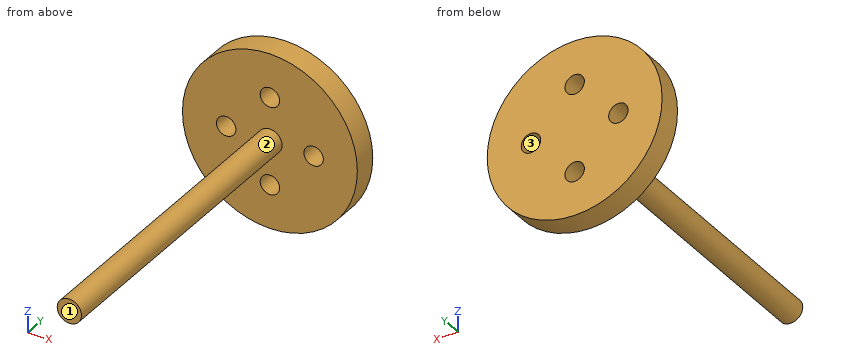
from build123d import *

# Parameters (mm, degrees)
SKETCH_1_R      = 18
SKETCH_1_R_2    = 2
EXTRUDE_1_DEPTH = 5
SKETCH_2_R      = 2.5
EXTRUDE_2_DEPTH = 65


with BuildPart() as part:
    # 草图1 → 凸台-拉伸1 (new body)
    with BuildSketch(Plane(origin=(0, 0, 0), x_dir=(1, 0, 0), z_dir=(0, 1, 0))):
        with Locations(Location((0, 0, 0), (0, 0, 270))):
            Circle(SKETCH_1_R)
        with Locations(Location((0, 9, 0), (0, 0, 270))):
            Circle(SKETCH_1_R_2, mode=Mode.SUBTRACT)
        with Locations(Location((9, 0, 0), (0, 0, 270))):
            Circle(SKETCH_1_R_2, mode=Mode.SUBTRACT)
        with Locations(Location((-9, 0, 0), (0, 0, 270))):
            Circle(SKETCH_1_R_2, mode=Mode.SUBTRACT)
        with Locations(Location((0, -9, 0), (0, 0, 270))):
            Circle(SKETCH_1_R_2, mode=Mode.SUBTRACT)
    extrude(amount=EXTRUDE_1_DEPTH)

    # 草图2 → 凸台-拉伸2 (add)
    with BuildSketch(Plane.XZ):
        with Locations(Location((0, 0, 0), (0, 0, 90))):
            Circle(SKETCH_2_R)
    extrude(amount=EXTRUDE_2_DEPTH)


solid = part.part
Part model, mm, in its own coordinate system. Face numbers are marked on the shaded views. Coordinates: 2 decimals unless noted, no trailing zeros. Order: outer loops, then holes, each group sorted by start corner. A loop starts at its lowest first (then second) coordinate and runs counter-clockwise, first axis right, second up.
(1) Probe L1, parallel to X at y = 2.5, z = 0; L2, parallel to X at y = -19.5, z = -1.5; L3, parallel to Y at x = -5.5, z = -11.5. List the from-to ranges inside material, lowest first.
Check sheet entries:
L1: x = -18 to -11, -7 to 7, 11 to 18
L2: x = -2 to 2
L3: y = 0 to 5
(2) Pull direction Z, two halves, no side cores. Call the marked faces 1, 2 and 3: pulls with the +Z half, pulls with the -Z half, needs draft (parallel to the pull), parting line crosses it, or undercut.
Check sheet entries:
face 1: needs draft
face 2: parting line crosses it
face 3: undercut
(3) Slice it at B-B, the plane x = 0. Write the cut outline in (y, z), and give its area (3 significant figures).
Check sheet entries:
outline: (-65, -2.5) - (0, -2.5) - (0, -7) - (5, -7) - (5, 7) - (0, 7) - (0, 2.5) - (-65, 2.5) - close; (0, -18) - (5, -18) - (5, -11) - (0, -11) - close; (0, 11) - (5, 11) - (5, 18) - (0, 18) - close
area: 465 mm2
(4) Slice it at C-C, the plane z = -9. Write the cut outline in (x, y).
Check sheet entries:
outline: (-15.59, 0) - (-2, 0) - (-2, 5) - (-15.59, 5) - close; (2, 0) - (15.59, 0) - (15.59, 5) - (2, 5) - close
(5) Slice it at D-D, the plane x = 9. Write the cut outline in (y, z).
Check sheet entries:
outline: (0, -15.59) - (5, -15.59) - (5, -2) - (0, -2) - close; (0, 2) - (5, 2) - (5, 15.59) - (0, 15.59) - close
(6) Pin check, flat tips, straight feed: pin 1 Ø4.5 at (x, z) = (-9, 0) entering from +Y; pin 2 Ø8 at (y, z) = (-25.5, 1.5) entering from +X; pin 3 Ø3 at (x, y) = (-0.5, -24.5) entering from +Z. Stop position of each tip, or through.
Check sheet entries:
pin 1: stops at y = 5
pin 2: stops at x = 2.5
pin 3: stops at z = 2.5
(7) Slice it at A-A, the plane z = 0. Write the cut outline in (x, y), and give its area (3 significant figures).
Check sheet entries:
outline: (-18, 0) - (-11, 0) - (-11, 5) - (-18, 5) - close; (-7, 0) - (-2.5, 0) - (-2.5, -65) - (2.5, -65) - (2.5, 0) - (7, 0) - (7, 5) - (-7, 5) - close; (11, 0) - (18, 0) - (18, 5) - (11, 5) - close
area: 465 mm2
